```python
from build123d import *

# Parameters (mm, degrees)
F0_W     = 45
F0_H     = 30
F0_R     = 2.5
F1_DEPTH = 20
F2_R     = 2.5
F3_DEPTH = 45.001
F2_R_2   = 5.5
F4_DEPTH = 20
F5_SIZE  = 2.99999


# Not quite as in the source:
# - a fillet or chamfer is up to 0.001 mm smaller than in the source, because OpenCascade refuses the exact size


with BuildPart() as f1:
    # F0 (on Top) → F1 (new body)
    with BuildSketch(Plane.XY):
        Rectangle(F0_W, F0_H)
        with Locations((11.25, 7.5)):
            Circle(F0_R, mode=Mode.SUBTRACT)
    extrude(amount=F1_DEPTH)

    # F2 (on face) → F3 (cut, through all)
    with BuildSketch(Plane.YZ.offset(22.5)):
        with Locations((-7.5, 10)):
            Circle(F2_R)
    extrude(amount=-F3_DEPTH, mode=Mode.SUBTRACT)

    # F2 (on face) → F4 (cut)
    with BuildSketch(Plane.YZ.offset(22.5)):
        with Locations((-7.5, 10)):
            Circle(F2_R_2)
        with Locations((-7.5, 10)):
            Circle(F2_R, mode=Mode.SUBTRACT)
    extrude(amount=-F4_DEPTH, mode=Mode.SUBTRACT)

    # F5 (size 3 in the source; OpenCascade refuses exactly that, so slightly less here)
    f5_edges = [f1.edges().sort_by_distance(p)[0] for p in [
        (8.75, 7.5, 20),
        (2.5, -13, 10),
    ]]
    chamfer(f5_edges, length=F5_SIZE)


solid = f1.part
```
Design review of the part built by this model. Coordinates are the model's own, in mm. A direction names the side the tool comes from. Coordinates: 2 decimals unless noted, no trailing zeros. Write each loop counter-clockwise with the first axis right and the second up, starting at its lowest first coordinate (ties: lowest second). Pieces come first, ordered by that corner, then holes. Notation, with made-up numbers: M 82.25,73 L 136.25,73 A9 ccw 136.25,83 Z; hole C -12,43.5 d10. An arc over 180 degrees is marked long. Answer as a JSON object with one key per item and string values.
Item 1: Draft analysis for pull direction X (two halves, no side actions). For faces 1 (the cylindrical face through (10.71, 5.06, 8.38)), 2 (the flat face through (-22.5, 0, 10)), 3 (the conical face through (2.688, -8.083, 7.376)), state which applies: pulls with the +X half, pulls with the -X half, needs draft (parallel to the pull), parting line crosses it, or undercut.
Outcome:
{"face 1": "undercut", "face 2": "pulls with the -X half", "face 3": "pulls with the +X half"}
Item 2: Machinability: for faces 4 (the cylindrical face through (14.1, -5, 5.1)), 5 (the flat face through (22.5, 0, 10)), which of the approach directions +Z, -Z, +X, -X, +Y, -Y give a long, thin tool a straight path to every point of the face, cutting with its end or side? Answer none if there is none.
Outcome:
{"face 4": "+X", "face 5": "+Z, -Z, +X, +Y, -Y"}
Item 3: Wall thickness on probe 1 along Z at (x, y) = (13.25, -7.5); probe 2 along Z at (x, y) = (-10.25, -7.5); probe 3 along Y at (x, z) = (11.25, 6): over which ranges is each line inside the solid? List them lowest first.
Outcome:
{"probe 1": "0 to 4.5, 15.5 to 20", "probe 2": "0 to 7.5, 12.5 to 20", "probe 3": "-15 to -11.27, -3.73 to 5, 10 to 15"}
Item 4: Insertion check: pin 1 Ø4 at (y, z) = (-7.5, 10) entering from +X; pin 2 Ø4 at (y, z) = (-7.5, 11) entering from +X. Each pin has a flat end and moves straight along its axis. Give the tip position at first contact, or say it passes through.
Outcome:
{"pin 1": "through", "pin 2": "x = 3"}
Item 5: Add section D-D, the plane z = 18. Give the boundary of the cut face in (x, y), and give its area (3 significant figures).
Outcome:
{"outline": "M -22.5,-15 L 22.5,-15 L 22.5,15 L -22.5,15 Z; hole C 11.25,7.5 d7", "area": "1,310 mm²"}
Item 6: Add section A-A, the plane z = 10. State how many separate pieces and enclosed holes the cut face has, and give its area (3 significant figures).
Outcome:
{"separate pieces": "2", "enclosed holes": "1", "area": "994 mm²"}
Item 7: Add section C-C, the plane x = 17.5. Give the boundary of the cut face in (y, z).
Outcome:
{"outline": "M -15,0 L 15,0 L 15,20 L -15,20 Z; hole C -7.5,10 d11"}
